Geometry: final body of the model. Coordinates: model frame, mm. A direction names the side the tool comes from. Give positions to 0.01 mm unless a question says otherwise; leave off trailing zeros. Write each loop counter-clockwise with the first axis right and the second up, starting at its lowest first coordinate (ties: lowest second). Pieces come first, ordered by that corner, then holes. Notation, with made-up numbers: (80, -28.75) -> (116, -28.75) arc R7 cw to (116, -21.75) -> close; hole circle Ø10 at (31, -20.75). An arc over 180 degrees is marked (long way). Use CSV: the item, a comma, the result in double quotes. Start each with the question number.
1) Section C-C (y = 23). Output: boundary loops of the cut face in (x, z) (3 decimals).
2) Section B-B (x = 57). Output: boundary loops of the cut face in (y, z) (1 decimal), plus the area to 3 significant figures.
3) Contact query for flat-ended pins moving along their axis: P1, Ø4, axis at y = 40.259, z = 11.811, coming from the -X side; P2, Ø4.5, axis at y = 40.259, z = -11.811, coming from the -X side; P3, Ø1.5, axis at x = 31, z = 34, coming from the +Y side. Output: stop coordinate, or through.
4) Section D-D (x = 5). Output: boundary loops of the cut face in (y, z) (3 decimals).
5) Section A-A (z = -30.5). Output: boundary loops of the cut face in (x, y).
6) Draft query along Z for faces 1 (the face through (53.975, 40, 12)), 2 (the face through (63.5, 40, 1)), 3 (the face through (58.8, 39.35, 9.61)), 4 (the face through (31, 24, 66.675)). Return one class per face: pulls with the +Z half, pulls with the -Z half, needs draft (parallel to the pull), parting line crosses it, or undercut.
7) Material intervals for line 1 (X direction, y = 22, z = 42.5); line 2 (Y direction, x = 59.5, z = -10); line 3 (X direction, y = 37.5, z = 15.5), sorted ascending. Write a range as [from, to].
8) Set-up query: faces 5 (the face through (50.8, 13, 1)), 6 (the face through (31, 24, -66.675)), 7 (the face through (58.8, 39.35, -14.01)). Return all of +Z, -Z, +X, -X, +Y, -Y with unobstructed straight access to the full face (end or side cutting, diameter ignored); none if empty.
```python
from build123d import *

# Parameters (mm, degrees)
SKETCH1_W           = 50.8
SKETCH1_H           = 26.576651581
BOSS_EXTRUDE1_DEPTH = 66.675
SKETCH3_R           = 2.38125
CUT_EXTRUDE1_DEPTH  = 9.525


with BuildPart() as part:
    # Sketch1 → Boss-Extrude1 (new body, symmetric)
    with BuildSketch(Plane.XY):
        with Locations((25.4, 13.288325791)):
            Rectangle(SKETCH1_W, SKETCH1_H)
        Polygon((34.697045256, 46.609), (0, 26.576651581), (50.8, 26.576651581), (63.5, 33.909), (63.5, 46.609), align=None)
    extrude(amount=BOSS_EXTRUDE1_DEPTH, both=True)

    # Sketch3 → Cut-Extrude1 (cut)
    with BuildSketch(Plane(origin=(63.5, 0, 0), x_dir=(0, 0, -1), z_dir=(1, 0, 0))):
        with Locations((-11.811, 40.259)):
            Circle(SKETCH3_R)
        with Locations((11.811, 40.259)):
            Circle(SKETCH3_R)
    extrude(amount=-CUT_EXTRUDE1_DEPTH, mode=Mode.SUBTRACT)


solid = part.part
```
Answers follow:
1,outline,"(0, -66.675) -> (50.8, -66.675) -> (50.8, 66.675) -> (0, 66.675) -> close"
2,outline,"(30.2, -66.7) -> (46.6, -66.7) -> (46.6, 66.7) -> (30.2, 66.7) -> close; hole circle Ø4.8 at (40.3, -11.8); hole circle Ø4.8 at (40.3, 11.8)"
2,area,"2,160 mm^2"
3,P1,"stops at x = 20.23"
3,P2,"stops at x = 19.8"
3,P3,"stops at y = 44.91"
4,outline,"(0, -66.675) -> (29.463, -66.675) -> (29.463, 66.675) -> (0, 66.675) -> close"
5,outline,"(0, 0) -> (50.8, 0) -> (50.8, 26.58) -> (63.5, 33.91) -> (63.5, 46.61) -> (34.7, 46.61) -> (0, 26.58) -> close"
6,face 1,"undercut"
6,face 2,"needs draft"
6,face 3,"undercut"
6,face 4,"pulls with the +Z half"
7,line 1,"x = [0, 50.8]"
7,line 2,"y = [31.6, 38.71], [41.81, 46.61]"
7,line 3,"x = [18.92, 63.5]"
8,face 5,"+Z, -Z, +X, -Y"
8,face 6,"-Z, +X, -X, +Y, -Y"
8,face 7,"+X"
